Could you check a few things on this model? Use its own coordinates, in mm. Coordinates: 2 decimals unless noted, no trailing zeros. Write each loop counter-clockwise with the first axis right and the second up, starting at its lowest first coordinate (ties: lowest second). Pieces come first, ordered by that corner, then holes. Notation, with made-up numbers: (88, -25.75) - (110, -25.75) arc R24 cw to (110, 5.25) - close; hole circle Ø8 at (-34, 69). An arc over 180 degrees is marked (long way). Answer as a JSON object with one key per item and string values. Group by question number.
1) Will these pins go through, and if not, where does the flat tip stop? pin 1 Ø0.8 at (x, z) = (1228, 1) entering from -Y; pin 2 Ø0.5 at (x, z) = (1266, 1.5) entering from +Y; pin 3 Ø0.6 at (x, z) = (1230, 1) entering from +Y.
2) Please list where these lines run through material, in increasing order: line 1 along Y through (x, z) = (1243.5, 0.3); line 2 along X through (y, z) = (477, 1.3); line 3 along Y through (x, z) = (1251, 0.4).
3) If we section it at D-D (x = 1270): Write out the boundary of the cut face in (y, z), plus the area to 3 significant figures.
4) If we section it at A-A (y = 466): Write out the boundary of the cut face in (x, z), plus the area to 3 significant figures.
5) If we section it at B-B (x = 1260): Write out the boundary of the cut face in (y, z), plus the area to 3 significant figures.
6) If we section it at C-C (y = 457): Write out the boundary of the cut face in (x, z), plus the area to 3 significant figures.
```python
from build123d import *

# Parameters (mm, degrees)
EXTRUDE_1_DEPTH = 2


with BuildPart() as part:
    # Model → 凸台-拉伸1 (new body)
    with BuildSketch(Plane.XY):
        Polygon((1228.50953615, 484.721569843), (1228.50953615, 467.721569843), (1227.00953615, 467.721569843), (1227.00953615, 457.721569843), (1228.50953615, 457.721569843), (1228.50953615, 442.721569843), (1233.50953615, 442.721569843), (1233.50953615, 439.721569843), (1245.50953615, 439.721569843), (1245.50953615, 437.721569843), (1238.50953615, 437.721569843), (1238.50953615, 435.721569843), (1248.50953615, 435.721569843), (1248.50953615, 437.721569843), (1253.50953615, 437.721569843), (1253.50953615, 435.721569843), (1263.50953615, 435.721569843), (1263.50953615, 437.721569843), (1256.50953615, 437.721569843), (1256.50953615, 439.721569843), (1268.50953615, 439.721569843), (1268.50953615, 442.721569843), (1273.50953615, 442.721569843), (1273.50953615, 457.721569843), (1275.00953615, 457.721569843), (1275.00953615, 467.721569843), (1273.50953615, 467.721569843), (1273.50953615, 484.721569843), (1268.50953615, 484.721569843), (1268.50953615, 485.721569843), (1256.50953615, 485.721569843), (1256.50953615, 487.721569843), (1263.50953615, 487.721569843), (1263.50953615, 490.721569843), (1253.50953615, 490.721569843), (1253.50953615, 487.721569843), (1248.50953615, 487.721569843), (1248.50953615, 490.721569843), (1238.50953615, 490.721569843), (1238.50953615, 487.721569843), (1245.50953615, 487.721569843), (1245.50953615, 485.721569843), (1233.50953615, 485.721569843), (1233.50953615, 484.721569843), align=None)
        with BuildLine():
            Line((1235.50953615, 479.721569843), (1236.50953615, 479.721569843))
            ThreePointArc((1236.50953615, 479.721569843), (1237.923749713, 480.307356281), (1238.50953615, 481.721569843))
            Line((1238.50953615, 481.721569843), (1238.50953615, 482.721569843))
            Line((1238.50953615, 482.721569843), (1263.50953615, 482.721569843))
            Line((1263.50953615, 482.721569843), (1263.50953615, 481.721569843))
            ThreePointArc((1263.50953615, 481.721569843), (1264.095322588, 480.307356281), (1265.50953615, 479.721569843))
            Line((1265.50953615, 479.721569843), (1266.50953615, 479.721569843))
            ThreePointArc((1266.50953615, 479.721569843), (1267.923749713, 479.135783405), (1268.50953615, 477.721569843))
            Line((1268.50953615, 477.721569843), (1268.50953615, 449.721569843))
            ThreePointArc((1268.50953615, 449.721569843), (1267.923749713, 448.307356281), (1266.50953615, 447.721569843))
            Line((1266.50953615, 447.721569843), (1265.50953615, 447.721569843))
            ThreePointArc((1265.50953615, 447.721569843), (1264.095322588, 447.135783405), (1263.50953615, 445.721569843))
            Line((1263.50953615, 445.721569843), (1263.50953615, 444.721569843))
            ThreePointArc((1263.50953615, 444.721569843), (1262.923749713, 443.307356281), (1261.50953615, 442.721569843))
            Line((1261.50953615, 442.721569843), (1240.50953615, 442.721569843))
            ThreePointArc((1240.50953615, 442.721569843), (1239.095322588, 443.307356281), (1238.50953615, 444.721569843))
            Line((1238.50953615, 444.721569843), (1238.50953615, 445.721569843))
            ThreePointArc((1238.50953615, 445.721569843), (1237.923749713, 447.135783405), (1236.50953615, 447.721569843))
            Line((1236.50953615, 447.721569843), (1235.50953615, 447.721569843))
            ThreePointArc((1235.50953615, 447.721569843), (1234.095322588, 448.307356281), (1233.50953615, 449.721569843))
            Line((1233.50953615, 449.721569843), (1233.50953615, 477.721569843))
            ThreePointArc((1233.50953615, 477.721569843), (1234.095322588, 479.135783405), (1235.50953615, 479.721569843))
        make_face(mode=Mode.SUBTRACT)
    extrude(amount=EXTRUDE_1_DEPTH)


solid = part.part
```
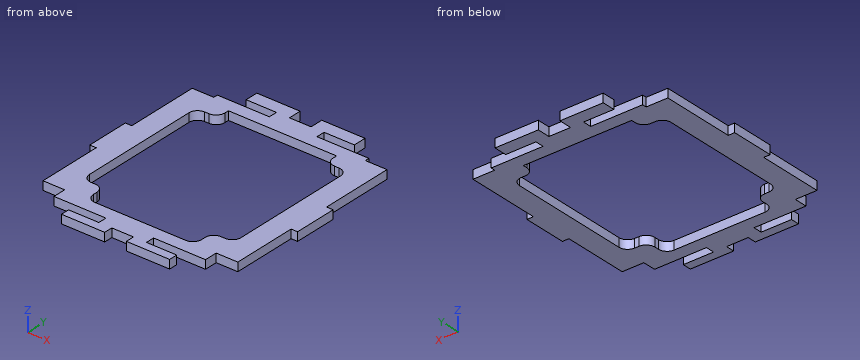
Here are the results:
{
 "1": {"pin 1": "stops at y = 457.72", "pin 2": "stops at y = 485.72", "pin 3": "stops at y = 484.72"},
 "2": {"line 1": "y = 435.72 to 437.72, 439.72 to 442.72, 482.72 to 485.72, 487.72 to 490.72", "line 2": "x = 1228.51 to 1233.51, 1268.51 to 1273.51", "line 3": "y = 437.72 to 442.72, 482.72 to 487.72"},
 "3": {"outline": "(442.72, 0) - (484.72, 0) - (484.72, 2) - (442.72, 2) - close", "area": "84.0 mm²"},
 "4": {"outline": "(1227.01, 0) - (1233.51, 0) - (1233.51, 2) - (1227.01, 2) - close; (1268.51, 0) - (1275.01, 0) - (1275.01, 2) - (1268.51, 2) - close", "area": "26.0 mm²"},
 "5": {"outline": "(435.72, 0) - (437.72, 0) - (437.72, 2) - (435.72, 2) - close; (439.72, 0) - (442.72, 0) - (442.72, 2) - (439.72, 2) - close; (482.72, 0) - (485.72, 0) - (485.72, 2) - (482.72, 2) - close; (487.72, 0) - (490.72, 0) - (490.72, 2) - (487.72, 2) - close", "area": "22.0 mm²"},
 "6": {"outline": "(1228.51, 0) - (1233.51, 0) - (1233.51, 2) - (1228.51, 2) - close; (1268.51, 0) - (1273.51, 0) - (1273.51, 2) - (1268.51, 2) - close", "area": "20.0 mm²"}
}
